Build history of the part. All positions in model axes, mm. A direction names the side the tool comes from. Coordinates: 2 decimals unless noted, no trailing zeros. Loops run counter-clockwise (first coordinate to the right, second up) from the corner with the lowest first, then second, coordinate; pieces in that order, holes last.
Item 1: Drill centre lines: line 1 along X through (y, z) = (-5370.5, -6); line 2 along Y through (x, z) = (-422.5, -12.75) (3 decimals); line 3 along Y through (x, z) = (-194, -14.25) (3 decimals). Where is each one in solid material? Low to high.
Item 2: Cut at B-B (x = -270). List the corners of the cut face in (y, z) (3 decimals), and give its area (3 significant figures).
Item 3: Flat gauge pin, fed straight in: pin 1 (8 mm diameter, centred on x = -398.17, z = -11.19, fed in from +Y). Where does the tip first touch, or does it go through?
Item 4: 3-axis set-ups, long thin cutter, end or side, ignore diameter. For faces 4 (the face through (-399, -5329.809, -5)), 5 (the face through (-238, -5502.275, -9)): which of +Z, -Z, +X, -X, +Y, -Y reach the whole face in a straight line?
Item 5: Cut at A-A (y = -5419.5). List the corners of the cut face in (x, z), and give its area (3 significant figures).
Item 6: Mould opens along Y. For faces 1 (the face through (-308.451, -5384, -9)), 2 (the face through (-238, -5449, 0)), 3 (the face through (-238, -5314.95, -9)) say: released by +Y, released by -Y, zero draft, split by the parting line, or undercut.
from build123d import *

# Parameters (mm, degrees)
HEADBOTTOMOUTLINE_W               = 740.41
HEADBOTTOMOUTLINE_H               = 187.325
HEADBOTTOMOUTLINE_THICKNESS_DEPTH = 17.78
SKETCH3_R                         = 1.5875
CUT_EXTRUDE1_DEPTH                = 17.78
SKETCH4_R                         = 5.08
CUT_EXTRUDE2_DEPTH                = 14.859


with BuildPart() as part:
    # HeadBottomOutline → HeadBottomOutline_Thickness (new body)
    with BuildSketch(Plane.XY):
        with Locations((-233.045, -5408.6125)):
            Rectangle(HEADBOTTOMOUTLINE_W, HEADBOTTOMOUTLINE_H)
    extrude(amount=-HEADBOTTOMOUTLINE_THICKNESS_DEPTH)

    # Sketch3 → Cut-Extrude1 (cut)
    with BuildSketch(Plane.XY):
        with Locations((-429.895, -5484.0124)):
            Circle(SKETCH3_R)
        with Locations((-379.095, -5484.0124)):
            Circle(SKETCH3_R)
        with Locations((-86.995, -5484.0124)):
            Circle(SKETCH3_R)
        with Locations((-36.195, -5484.0124)):
            Circle(SKETCH3_R)
        with BuildLine():
            Line((-308.45125, -5335.905), (-308.45125, -5433.695))
            ThreePointArc((-308.45125, -5433.695), (-307.52131403, -5435.94006403), (-305.27625, -5436.87))
            Line((-305.27625, -5436.87), (-160.81375, -5436.87))
            ThreePointArc((-160.81375, -5436.87), (-158.56868597, -5435.94006403), (-157.63875, -5433.695))
            Line((-157.63875, -5433.695), (-157.63875, -5335.905))
            ThreePointArc((-157.63875, -5335.905), (-158.56868597, -5333.65993597), (-160.81375, -5332.73))
            Line((-160.81375, -5332.73), (-305.27625, -5332.73))
            ThreePointArc((-305.27625, -5332.73), (-307.52131403, -5333.65993597), (-308.45125, -5335.905))
        make_face()
        with BuildLine():
            Line((-354.2665, -5334), (-354.2665, -5341.9375))
            ThreePointArc((-354.2665, -5341.9375), (-356.888919435, -5348.268580565), (-363.22, -5350.891))
            Line((-363.22, -5350.891), (-433.07, -5350.891))
            ThreePointArc((-433.07, -5350.891), (-439.401080565, -5348.268580565), (-442.0235, -5341.9375))
            Line((-442.0235, -5341.9375), (-442.0235, -5334))
            ThreePointArc((-442.0235, -5334), (-440.79598452, -5331.03651548), (-437.8325, -5329.809))
            Line((-437.8325, -5329.809), (-358.4575, -5329.809))
            ThreePointArc((-358.4575, -5329.809), (-355.49401548, -5331.03651548), (-354.2665, -5334))
        make_face()
        with BuildLine():
            Line((-102.87, -5350.891), (-33.02, -5350.891))
            ThreePointArc((-33.02, -5350.891), (-26.688919435, -5348.268580565), (-24.0665, -5341.9375))
            Line((-24.0665, -5341.9375), (-24.0665, -5334))
            ThreePointArc((-24.0665, -5334), (-25.29401548, -5331.03651548), (-28.2575, -5329.809))
            Line((-28.2575, -5329.809), (-107.6325, -5329.809))
            ThreePointArc((-107.6325, -5329.809), (-110.59598452, -5331.03651548), (-111.8235, -5334))
            Line((-111.8235, -5334), (-111.8235, -5341.9375))
            ThreePointArc((-111.8235, -5341.9375), (-109.201080565, -5348.268580565), (-102.87, -5350.891))
        make_face()
    extrude(amount=-CUT_EXTRUDE1_DEPTH, mode=Mode.SUBTRACT)

    # Sketch4 → Cut-Extrude2 (cut)
    with BuildSketch(Plane(origin=(0, -5314.95, 0), x_dir=(1, 0, 0), z_dir=(0, 1, 0))):
        with Locations((-67.9699936, 11.187303)):
            Circle(SKETCH4_R)
        with Locations((-398.1699936, 11.187303)):
            Circle(SKETCH4_R)
    extrude(amount=-CUT_EXTRUDE2_DEPTH, mode=Mode.SUBTRACT)


solid = part.part
Filled sheet:
1. line 1: x = -603.25 to -308.45, -157.64 to 137.16
1. line 2: y = -5502.275 to -5350.891, -5329.809 to -5314.95
1. line 3: y = -5502.275 to -5436.87, -5332.73 to -5314.95
2. outline: (-5502.275, -17.78) - (-5436.87, -17.78) - (-5436.87, 0) - (-5502.275, 0) - close; (-5332.73, -17.78) - (-5314.95, -17.78) - (-5314.95, 0) - (-5332.73, 0) - close
2. area: 1,480 mm2
3. pin 1: stops at y = -5350.89
4. face 4: +Z, -Z
4. face 5: +Z, -Z, +X, -X, -Y
5. outline: (-603.25, -17.78) - (-308.45, -17.78) - (-308.45, 0) - (-603.25, 0) - close; (-157.64, -17.78) - (137.16, -17.78) - (137.16, 0) - (-157.64, 0) - close
5. area: 10,500 mm2
6. face 1: undercut
6. face 2: zero draft
6. face 3: released by +Y
